Check sheet for the drawn part. Datum: minimum x, y, z corner. Units: mm. Round coordinates to 2 decimals unless told otherwise and drop trailing zeros. Write each loop counter-clockwise with the first axis right and the second up, starting at its lowest first coordinate (ties: lowest second). Pieces come first, ordered by that corner, then holes. Notation, with made-up numbers: (37, -40) - (72, -40) arc R35 cw to (72, -5) - close; hole circle Ø9 at (66, 51). An arc over 180 degrees is marked (long way). Answer as a JSON object with one key per item and string values. Group by question number.
1) Mould release check, pull along Z, two halves, no side actions. Record for the marked faces 1, 2 and 3: +Z half, -Z half, draft (parallel to the pull), parting line (faces both ways), or undercut.
2) Thickness scan on line 1 (Y direction, x = 14.7, z = 29.5); line 2 (Z direction, x = 1.5, y = 15.5); line 3 (Y direction, x = 10, z = 62). Record the ranges inside material, lowest first.
3) Section check A-A (y = 14.7). Enter the section's corners in (x, z).
4) Section check D-D (x = 10.25). Enter the section's corners in (y, z).
5) Section check C-C (z = 39.5). Enter the section's corners in (x, y).
6) Go/stop test with flat-tipped pins: pin 1 Ø5 at (x, z) = (4.5, 14.5) entering from +Y; pin 2 Ø1 at (x, z) = (21.5, 54.5) entering from +Y; pin 3 Ø1 at (y, z) = (7.5, 14) entering from +X; pin 4 Ø4.5 at (x, y) = (14.7, 14.7) entering from +Z. Record where each tip stops, or that it passes through.
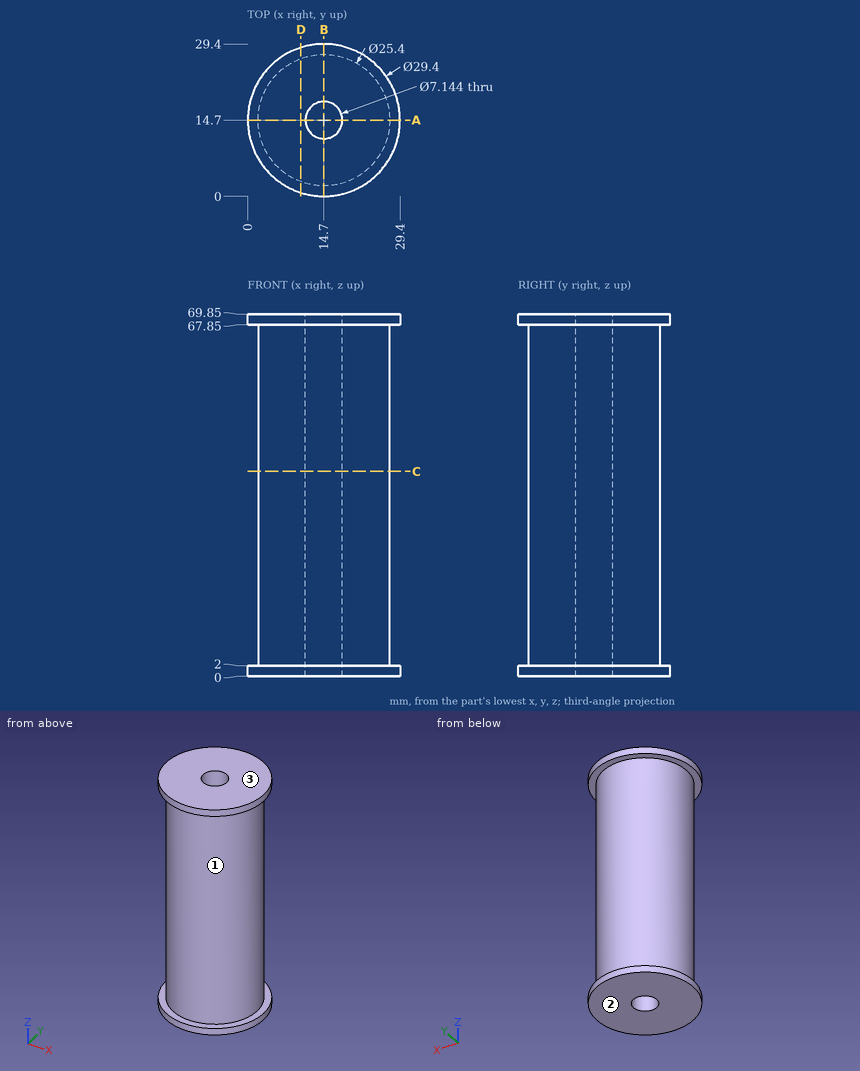
Returned:
{
 "1": {"face 1": "undercut", "face 2": "-Z half", "face 3": "+Z half"},
 "2": {"line 1": "2 to 11.13, 18.27 to 27.4", "line 2": "0 to 2, 67.85 to 69.85", "line 3": "2.9 to 26.5"},
 "3": {"outline": "(0, 0) - (11.13, 0) - (11.13, 69.85) - (0, 69.85) - (0, 67.85) - (2, 67.85) - (2, 2) - (0, 2) - close; (18.27, 0) - (29.4, 0) - (29.4, 2) - (27.4, 2) - (27.4, 67.85) - (29.4, 67.85) - (29.4, 69.85) - (18.27, 69.85) - close"},
 "4": {"outline": "(0.69, 0) - (28.71, 0) - (28.71, 2) - (26.59, 2) - (26.59, 67.85) - (28.71, 67.85) - (28.71, 69.85) - (0.69, 69.85) - (0.69, 67.85) - (2.81, 67.85) - (2.81, 2) - (0.69, 2) - close"},
 "5": {"outline": "circle Ø25.4 at (14.7, 14.7); hole circle Ø7.14 at (14.7, 14.7)"},
 "6": {"pin 1": "y = 24.8", "pin 2": "y = 25.73", "pin 3": "x = 25.49", "pin 4": "through"}
}
